Here's how the part is built. I have some questions about the finished solid (model axes, mm). A direction names the side the tool comes from. Coordinates: 2 decimals unless noted, no trailing zeros. Order: outer loops, then holes, each group sorted by start corner. A loop starts at its lowest first (then second) coordinate and runs counter-clockwise, first axis right, second up. Notation, with made-up numbers: (71.5, 71.5) - (113.5, 71.5) arc R14 cw to (113.5, 93.5) - close; hole circle Ø11 at (-36.5, 47). An arc over 180 degrees is marked (long way). Answer as CSV lines item,"result". Start each with the question number.
Q1. Thinking about a two-plate mould opening in X: for faces 1 (the face through (6, 12, 2)), 2 (the face through (-9, 15, 2)), 3 (the face through (45, -8, 2)), which applies, released by +X, released by -X, zero draft, split by the parting line, or undercut?
Q2. Suppose I cut it at C-C (x = 0). Please give me the cut outline in (y, z), then the cut area to 3 significant figures.
Q3. I need wall thicknesses on line 1 (X direction, y = -13.5, z = 63.5); line 2 (X direction, y = 0.25, z = -39); line 3 (Y direction, x = -7.5, z = -90). Which ranges of each line are inside material? Lowest first, please.
Q4. Suppose I cut it at A-A (x = 15). Please give me the cut outline in (y, z), then the cut area to 3 significant figures.
Q5. Suppose I cut it at B-B (z = 64). Count the separate pieces of the cut face and the enclosed holes in it, then the cut area to 3 significant figures.
Q6. For faces 4 (the face through (-7, 0, 2)), 5 (the face through (15, -15, 2)), which set-ups out of +Z, -Z, +X, -X, +Y, -Y let a thin tool reach every point of the face, with its end or its side?
Q7. For pin 1 Ø3 at (x, z) = (30, 50.5) entering from -Y, with a flat end and sliding along its axis, tell me the tip position at first contact or that it passes through.
from build123d import *

# Parameters (mm, degrees)
SALIENTE_EXTRUIR1_DEPTH = 115
REDONDEO1_R             = 1


with BuildPart() as part:
    # Croquis1 → Saliente-Extruir1 (new body, symmetric)
    with BuildSketch(Plane.XY):
        Polygon((-4.171572875, 7), (4.171572875, 7), (9.171572875, 12), (3, 12), (3, 15), (27, 15), (27, 12), (20.828427125, 12), (25.828427125, 7), (34.171572875, 7), (39.171572875, 12), (33, 12), (33, 15), (45, 15), (45, 3), (42, 3), (42, 9.171572875), (37, 4.171572875), (37, -4.171572875), (42, -9.171572875), (42, -3), (45, -3), (45, -15), (33, -15), (33, -12), (39.171572875, -12), (34.171572875, -7), (25.828427125, -7), (20.828427125, -12), (27, -12), (27, -15), (3, -15), (3, -12), (9.171572875, -12), (4.171572875, -7), (-4.171572875, -7), (-9.171572875, -12), (-3, -12), (-3, -15), (-15, -15), (-15, -3), (-12, -3), (-12, -9.171572875), (-7, -4.171572875), (-7, 4.171572875), (-12, 9.171572875), (-12, 3), (-15, 3), (-15, 15), (-3, 15), (-3, 12), (-9.171572875, 12), align=None)
        Polygon((7, 4.171572875), (7, -4.171572875), (12, -9.171572875), (12, -3), (18, -3), (18, -9.171572875), (23, -4.171572875), (23, 4.171572875), (18, 9.171572875), (18, 3), (12, 3), (12, 9.171572875), align=None, mode=Mode.SUBTRACT)
        with BuildLine():
            ThreePointArc((2.828427125, 2.828427125), (0, 4), (-2.828427125, 2.828427125))
            ThreePointArc((-2.828427125, 2.828427125), (-4, 0), (-2.828427125, -2.828427125))
            ThreePointArc((-2.828427125, -2.828427125), (0, -4), (2.828427125, -2.828427125))
            ThreePointArc((2.828427125, -2.828427125), (4, 0), (2.828427125, 2.828427125))
        make_face(mode=Mode.SUBTRACT)
        with BuildLine():
            ThreePointArc((32.828427125, 2.828427125), (34, 0), (32.828427125, -2.828427125))
            ThreePointArc((32.828427125, -2.828427125), (30, -4), (27.171572875, -2.828427125))
            ThreePointArc((27.171572875, -2.828427125), (26, 0), (27.171572875, 2.828427125))
            ThreePointArc((27.171572875, 2.828427125), (30, 4), (32.828427125, 2.828427125))
        make_face(mode=Mode.SUBTRACT)
    extrude(amount=SALIENTE_EXTRUIR1_DEPTH, both=True)

    # Redondeo1
    redondeo1_edges = [part.edges().sort_by_distance(p)[0] for p in [
        (-15, 15, 0),
        (45, 15, 0),
        (45, -15, 0),
        (-15, -15, 0),
    ]]
    fillet(redondeo1_edges, radius=REDONDEO1_R)


solid = part.part
Here are the results:
1,face 1,"undercut"
1,face 2,"zero draft"
1,face 3,"released by +X"
2,outline,"(-7, -115) - (-4, -115) - (-4, 115) - (-7, 115) - close; (4, -115) - (7, -115) - (7, 115) - (4, 115) - close"
2,area,"1,380 mm²"
3,line 1,"x = -15 to -3, 3 to 27, 33 to 45"
3,line 2,"x = -7 to -3.99, 3.99 to 7, 23 to 26.01, 33.99 to 37"
3,line 3,"y = -15 to -12, -10.33 to -4.67, 4.67 to 10.33, 12 to 15"
4,outline,"(-15, -115) - (-3, -115) - (-3, 115) - (-15, 115) - close; (3, -115) - (15, -115) - (15, 115) - (3, 115) - close"
4,area,"5,520 mm²"
5,separate pieces,"1"
5,enclosed holes,"3"
5,area,"1,020 mm²"
6,face 4,"+Z, -Z"
6,face 5,"+Z, -Z, +X, -X, -Y"
7,pin 1,"stops at y = -7"
